from build123d import *

# Parameters (mm, degrees)
F0_W     = 59
F0_H     = 50
F1_DEPTH = 12.5
F3_R     = 12.5
F4_DEPTH = 7


with BuildPart() as f1:
    # F0 (on Front) → F1 (new body, symmetric)
    with BuildSketch(Plane.XZ):
        Rectangle(F0_W, F0_H)
    extrude(amount=F1_DEPTH, both=True)

    # F3 (on face) → F4 (join)
    with BuildSketch(Plane.XZ.offset(12.5)):
        with Locations((12.0948115364, 5.6871213019)):
            Circle(F3_R)
    extrude(amount=F4_DEPTH)


solid = f1.part
Could you check a few things on this model? Use its own coordinates, in mm. A direction names the side the tool comes from. Coordinates: 2 decimals unless noted, no trailing zeros. Order: outer loops, then holes, each group sorted by start corner. A loop starts at its lowest first (then second) coordinate and runs counter-clockwise, first axis right, second up. Notation, with made-up numbers: (53.5, 10) -> (101.5, 10) arc R22 ccw to (101.5, 42) -> close; hole circle Ø5 at (-38, -1.75). An arc over 180 degrees is marked (long way). One line per item, written item: value. Start each with the question number.
1) I'm going to push a flat-ended pin straight in: pin 1 (6 mm diameter, centred on x = -13.5, z = -12, fed in from -Y). Where does the tip first touch, or does it pass through?
2) Imagine slicing it at D-D on y = -13.5. List the corners of the cut face in (x, z) for me.
3) Which directions (+Z, -Z, +X, -X, +Y, -Y) give clear straight access to the entire face, cutting with the end or side of a thin tool? Please do faces 1 (the cylindrical face through (2.175, -15.951, -1.919)), 2 (the flat face through (-29.5, 0, 0)).
4) If I drill on L1, parallel to Y at x = 27.5, z = -13; L2, parallel to Z at x = 8, y = -17, over which ranges is the centre line in solid material (lowest first)? Write a range as [from, to].
5) Imagine slicing it at A-A on z = -4. List the corners of the cut face in (x, y) for me.
6) Imagine slicing it at B-B on x = 11. List the corners of the cut face in (y, z) for me, plus the area to 3 significant figures.
7) Imagine slicing it at C-C on x = -13. List the corners of the cut face in (y, z) for me, plus the area to 3 significant figures.
Answer list:
1. pin 1: stops at y = -12.5
2. outline: circle Ø25 at (12.09, 5.69)
3. face 1: -Y
3. face 2: +Z, -Z, -X, +Y, -Y
4. L1: y = [-12.5, 12.5]
4. L2: z = [-6.12, 17.5]
5. outline: (-29.5, -12.5) -> (4.19, -12.5) -> (4.19, -19.5) -> (19.99, -19.5) -> (19.99, -12.5) -> (29.5, -12.5) -> (29.5, 12.5) -> (-29.5, 12.5) -> close
6. outline: (-19.5, -6.76) -> (-12.5, -6.76) -> (-12.5, -25) -> (12.5, -25) -> (12.5, 25) -> (-12.5, 25) -> (-12.5, 18.14) -> (-19.5, 18.14) -> close
6. area: 1,420 mm2
7. outline: (-12.5, -25) -> (12.5, -25) -> (12.5, 25) -> (-12.5, 25) -> close
7. area: 1,250 mm2
